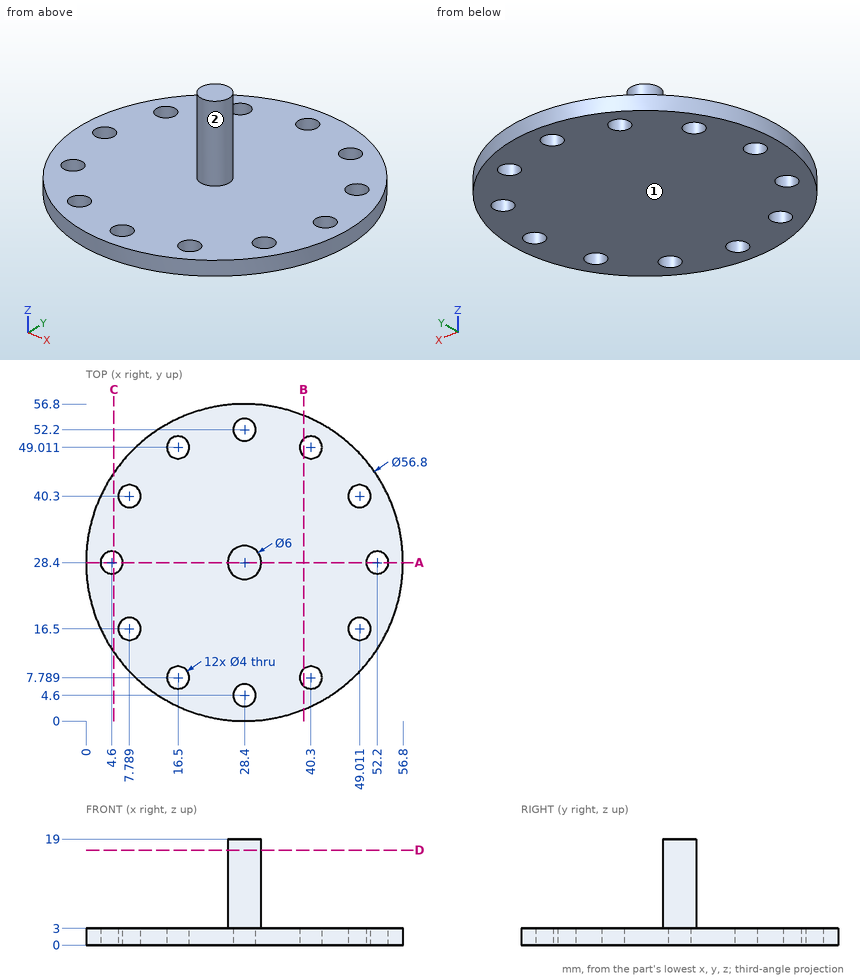
The drawing under review shows one solid part. Ordinate dimensions are in mm from its lowest x, y, z. A direction names the side the tool comes from. Round coordinates to 2 decimals unless told otherwise and drop trailing zeros. Write each loop counter-clockwise with the first axis right and the second up, starting at its lowest first coordinate (ties: lowest second). Pieces come first, ordered by that corner, then holes. Notation, with made-up numbers: (-1.75, 37) - (50.25, 37) arc R9 ccw to (50.25, 45) - close; hole circle Ø4 at (-20.75, 28.5). An arc over 180 degrees is marked (long way). One line per question, with ' | ' between items.
Item 1: Add section C-C, the plane x = 5. Give the boundary of the cut face in (y, z).
Resolved:
outline: (12.31, 0) - (26.44, 0) - (26.44, 3) - (12.31, 3) - close; (30.36, 0) - (44.49, 0) - (44.49, 3) - (30.36, 3) - close
Item 2: Add section B-B, the plane x = 39. Give the boundary of the cut face in (y, z), then the cut area to 3 significant figures.
Resolved:
outline: (2.05, 0) - (6.27, 0) - (6.27, 3) - (2.05, 3) - close; (9.31, 0) - (47.49, 0) - (47.49, 3) - (9.31, 3) - close; (50.53, 0) - (54.75, 0) - (54.75, 3) - (50.53, 3) - close | area: 140 mm2
Item 3: For the marked faces 1 and 2, list the 3-axis set-ups (+Z, -Z, +X, -X, +Y, -Y) from which the entire face can be reached by the end or side of a thin tool; tool diameter is ignored.
Resolved:
face 1: -Z, +X, -X, +Y, -Y | face 2: +Z
Item 4: Add section D-D, the plane z = 17. Give the boundary of the cut face in (x, y), then the cut area to 3 significant figures.
Resolved:
outline: circle Ø6 at (28.4, 28.4) | area: 28.3 mm2
Item 5: To check wall thickness, follow probe 1 along Y at (x, z) = (16.5, 1.55); probe 2 along Z at (x, y) = (6, 12); probe 3 along Y at (x, z) = (4.6, 1.1) (1 decimal). State the ranges of each line that lie inside material, in increasing order.
Resolved:
probe 1: y = 2.61 to 5.79, 9.79 to 47.01, 51.01 to 54.19 | probe 2: z = 0 to 3 | probe 3: y = 12.9 to 26.4, 30.4 to 43.9
Item 6: Add section A-A, the plane y = 28.4. Give the boundary of the cut face in (x, z).
Resolved:
outline: (0, 0) - (2.6, 0) - (2.6, 3) - (0, 3) - close; (6.6, 0) - (50.2, 0) - (50.2, 3) - (31.4, 3) - (31.4, 19) - (25.4, 19) - (25.4, 3) - (6.6, 3) - close; (54.2, 0) - (56.8, 0) - (56.8, 3) - (54.2, 3) - close
Item 7: For P1, Ø17, axis at x = 35, y = 17, coming from the +Z side; P2, Ø8, axis at y = 49.5, z = 5.5, coming from the -X side (1 decimal), all flat-tipped, find the tip position at first contact; note any pin that passes through.
Resolved:
P1: stops at z = 3 | P2: stops at x = 6.4
